Source: three-view drawing plus pictorial views. Frame: mm from the lowest corner of the part. Coordinates: 2 decimals unless noted, no trailing zeros. Write each loop counter-clockwise with the first axis right and the second up, starting at its lowest first coordinate (ties: lowest second). Pieces come first, ordered by that corner, then holes. Notation, with made-up numbers: (35.5, -24) - (92.5, -24) arc R6 cw to (92.5, -13) - close; hole circle Ø6 at (-25, -21). An arc over 180 degrees is marked (long way). Put each result on its own line as item: value.
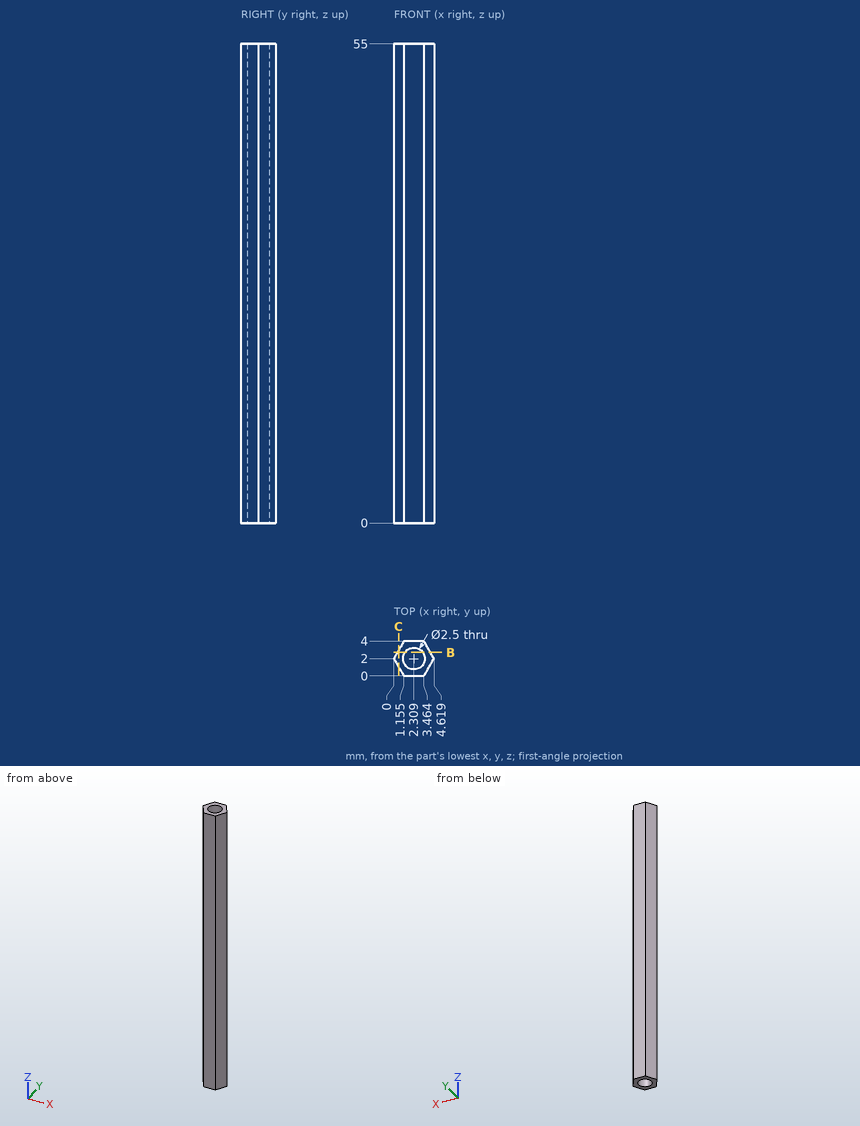
1. Section query B-B (y = 2.7). Return loops of the section in (x, z) (1 decimal).
Answer below:
outline: (0.4, 0) - (1.3, 0) - (1.3, 55) - (0.4, 55) - close; (3.3, 0) - (4.2, 0) - (4.2, 55) - (3.3, 55) - close
2. Section query C-C (x = 0.55). Return loops of the section in (y, z), then the cut area to 3 significant figures.
Answer below:
outline: (1.05, 0) - (2.95, 0) - (2.95, 55) - (1.05, 55) - close
area: 105 mm²
3. Ray query, probe 1 along X at (y, z) = (2, 13); probe 2 along Y at (x, z) = (2.2, 38.5) (1 decimal); probe 3 along Y at (x, z) = (3.35, 38.5) (1 decimal). Return the intervals inside material, ascending. Write a range as from..to.
Answer below:
probe 1: x = 0..1.06, 3.56..4.62
probe 2: y = 0..0.8, 3.2..4
probe 3: y = 0..1.3, 2.7..4
